Can you work these out from the drawing? Everything is in mm from the part's minimum corner. A direction names the side the tool comes from. Coordinates: 2 decimals unless noted, no trailing zeros. Write each loop counter-clockwise with the first axis right and the second up, starting at its lowest first coordinate (ties: lowest second). Pieces come first, ordered by that corner, then holes. Notation, with made-up numbers: (23.25, -11) -> (75.25, -11) arc R25 ccw to (75.25, 12) -> close; hole circle Ø3 at (-22.5, 18). An arc over 180 degrees is marked (long way). Answer as CSV lines item,"result". Start each with the question number.
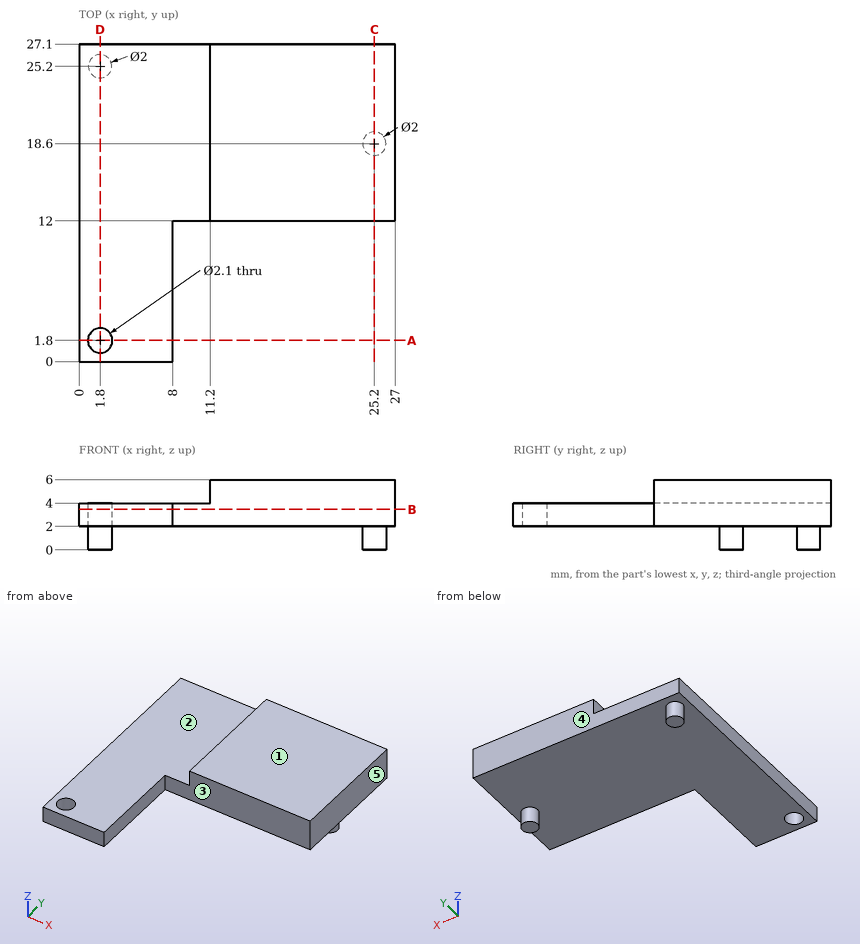
Q1. For pin 1 (3.5 mm diameter, centred on x = 1.8, y = 1.8, fed in from -Z); pin 2 (5.5 mm diameter, centred on x = 6.5, y = 17, fed in from +Z); pin 3 (2 mm diameter, centred on y = 8, z = 3, fed in from +X), each with a flat end and sliding along its axis, tell me the tip position at first contact or that it passes through.
Q2. I need wall thicknesses on L1, parallel to Y at x = 1.8, z = 3.5; L2, parallel to Z at x = 21.5, y = 13.25; L3, parallel to Y at x = 22, z = 4.2. Which ranges of each line are inside material? Lowest first, please.
Q3. Imagine slicing it at D-D (x = 1.8). Write out the boundary of the cut face in (y, z), then the cut area to 3 significant figures.
Q4. Imagine slicing it at B-B (z = 3.45). Write out the boundary of the cut face in (x, y), then the cut area to 3 significant figures.
Q5. Imagine slicing it at A-A (y = 1.8). Write out the boundary of the cut face in (x, z), then the cut area to 3 significant figures.
Q6. Imagine slicing it at C-C (x = 25.2). Write out the boundary of the cut face in (y, z).
Q7. If we mould it in two halves opening along X, with no side actions, what happens to the marked faces 4 and 5? For each: released by +X, released by -X, zero draft, split by the parting line, or undercut.
Q8. Which directions (+Z, -Z, +X, -X, +Y, -Y) give clear straight access to the entire face, cutting with the end or side of a thin tool? Please do the marked faces 1, 2 and 3.
Entries:
1,pin 1,"z = 2"
1,pin 2,"z = 4"
1,pin 3,"x = 8"
2,L1,"0 to 0.75, 2.85 to 27.1"
2,L2,"2 to 6"
2,L3,"12 to 27.1"
3,outline,"(0, 2) -> (0.75, 2) -> (0.75, 4) -> (0, 4) -> close; (2.85, 2) -> (24.2, 2) -> (24.2, 0) -> (26.2, 0) -> (26.2, 2) -> (27.1, 2) -> (27.1, 4) -> (2.85, 4) -> close"
3,area,"54.0 mm2"
4,outline,"(0, 0) -> (8, 0) -> (8, 12) -> (27, 12) -> (27, 27.1) -> (0, 27.1) -> close; hole circle Ø2.1 at (1.8, 1.8)"
4,area,"500 mm2"
5,outline,"(0, 2) -> (0.75, 2) -> (0.75, 4) -> (0, 4) -> close; (2.85, 2) -> (8, 2) -> (8, 4) -> (2.85, 4) -> close"
5,area,"11.8 mm2"
6,outline,"(12, 2) -> (17.6, 2) -> (17.6, 0) -> (19.6, 0) -> (19.6, 2) -> (27.1, 2) -> (27.1, 6) -> (12, 6) -> close"
7,face 4,"zero draft"
7,face 5,"released by +X"
8,face 1,"+Z, +X, -X, +Y, -Y"
8,face 2,"+Z, -X, +Y, -Y"
8,face 3,"+Z, -Z, +X, -Y"
